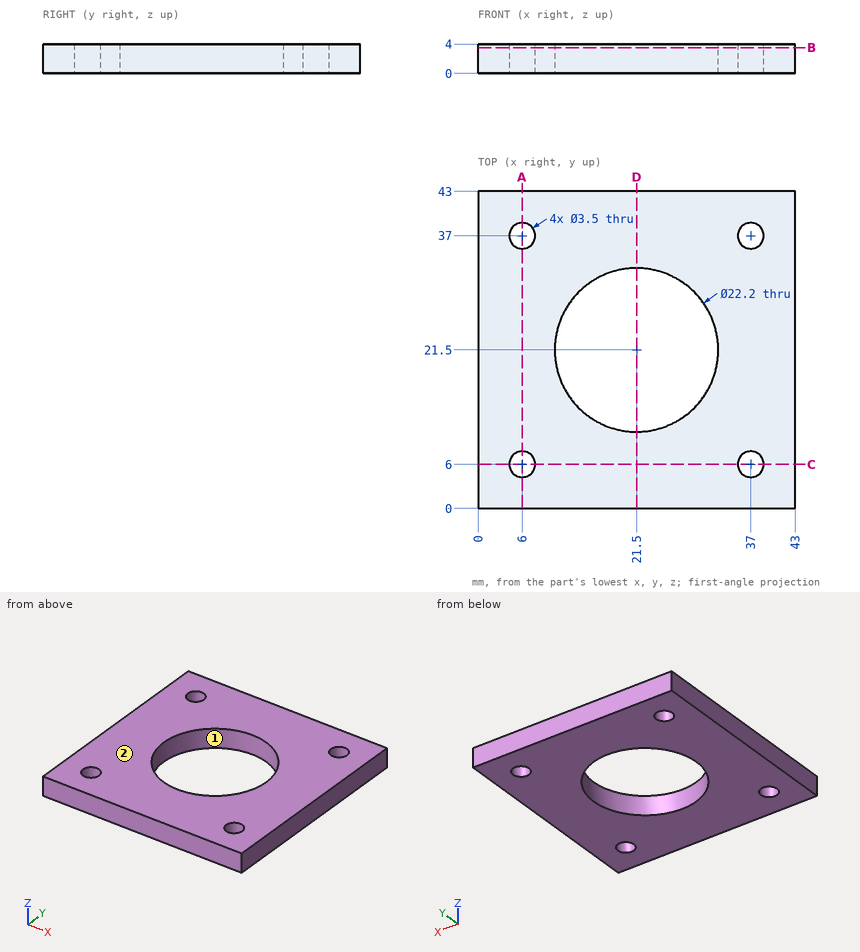
Drawing for the job (mm, zero at the part's lowest x, y, z). Round coordinates to 2 decimals unless told otherwise and drop trailing zeros. Write each loop counter-clockwise with the first axis right and the second up, starting at its lowest first coordinate (ties: lowest second). Pieces come first, ordered by that corner, then holes. Notation, with made-up numbers: (29, 10.5) - (83, 10.5) arc R37 ccw to (83, 49.5) - close; hole circle Ø4 at (62, -27.75). An arc over 180 degrees is marked (long way). Return JSON: item names as keys, results as strings. Group by question number.
Item 1: Flat gauge pin, fed straight in: pin 1 Ø3 at (x, y) = (37, 37) entering from -Z. Where does the tip first touch, or does it go through?
Item 2: Mould opens along X. For the marked faces 1 and 2 say: +X half, -X half, draft (parallel to the pull), parting line (faces both ways), or undercut.
Item 3: Band-saw the part on D-D on x = 21.5. List the corners of the cut face in (y, z).
Item 4: Band-saw the part on B-B on z = 3.5. List the corners of the cut face in (x, y).
Item 5: Probe probe 1 along Y at (x, z) = (6, 2.7); probe 2 along Y at (x, z) = (21.5, 3.15); probe 3 along Y at (x, z) = (5, 0.9). List the from-to ranges inside material, lowest first.
Item 6: Band-saw the part on A-A on x = 6. List the corners of the cut face in (y, z).
Resolved:
{
 "1": {"pin 1": "passes through"},
 "2": {"face 1": "undercut", "face 2": "draft"},
 "3": {"outline": "(0, 0) - (10.4, 0) - (10.4, 4) - (0, 4) - close; (32.6, 0) - (43, 0) - (43, 4) - (32.6, 4) - close"},
 "4": {"outline": "(0, 0) - (43, 0) - (43, 43) - (0, 43) - close; hole circle Ø3.5 at (6, 6); hole circle Ø3.5 at (6, 37); hole circle Ø22.2 at (21.5, 21.5); hole circle Ø3.5 at (37, 6); hole circle Ø3.5 at (37, 37)"},
 "5": {"probe 1": "y = 0 to 4.25, 7.75 to 35.25, 38.75 to 43", "probe 2": "y = 0 to 10.4, 32.6 to 43", "probe 3": "y = 0 to 4.56, 7.44 to 35.56, 38.44 to 43"},
 "6": {"outline": "(0, 0) - (4.25, 0) - (4.25, 4) - (0, 4) - close; (7.75, 0) - (35.25, 0) - (35.25, 4) - (7.75, 4) - close; (38.75, 0) - (43, 0) - (43, 4) - (38.75, 4) - close"}
}
